The figure shows three views and two pictorial views of one solid part (mm, origin at its lowest corner). Answer the questions. Coordinates: 2 decimals unless noted, no trailing zeros. Loops run counter-clockwise (first coordinate to the right, second up) from the corner with the lowest first, then second, coordinate; pieces in that order, holes last. Notation, with made-up numbers: M 11.25,36 L 15.25,36 A7 ccw 15.25,45 Z; hole C 51.5,45.25 d4. An arc over 180 degrees is marked long. One line per item, written item: value. Start each with the question number.
1. The part is cut by section D-D (y = 4). Write down the section's boundary in (x, z) (1 decimal).
2. Consider probe 1 along Z at (x, y) = (36.5, 9.5); probe 2 along Z at (x, y) = (44, 1.5); probe 3 along Y at (x, z) = (46, 16.75). Determine where each line is inside the solid, lowest interval first.
3. The part is cut by section A-A (z = 7.5). Write down the section's boundary in (x, y).
4. Determine the mould class of the marked faces 1, 2, 3 and 4 for opening direction Z: +Z half, -Z half, draft (parallel to the pull), parting line (faces both ways), or undercut.
5. The part is cut by section B-B (x = 21.5). Write down the section's boundary in (y, z).
6. Flat-ended cylindrical pins translate along their axes: pin 1 (4 mm diameter, centred on x = 43.97, z = 7.5, fed in from +Y); pin 2 (5 mm diameter, centred on y = 8, z = 21, fed in from -X); pin 3 (2 mm diameter, centred on y = 3, z = 25.5, fed in from -X) (1 decimal); pin 4 (2.5 mm diameter, centred on x = 37.67, z = 7.5, fed in from -Y). Find the tip coordinate at first contact, or state that the pin passes through.
7. The part is cut by section C-C (z = 12.5). Write down the section's boundary in (x, y).
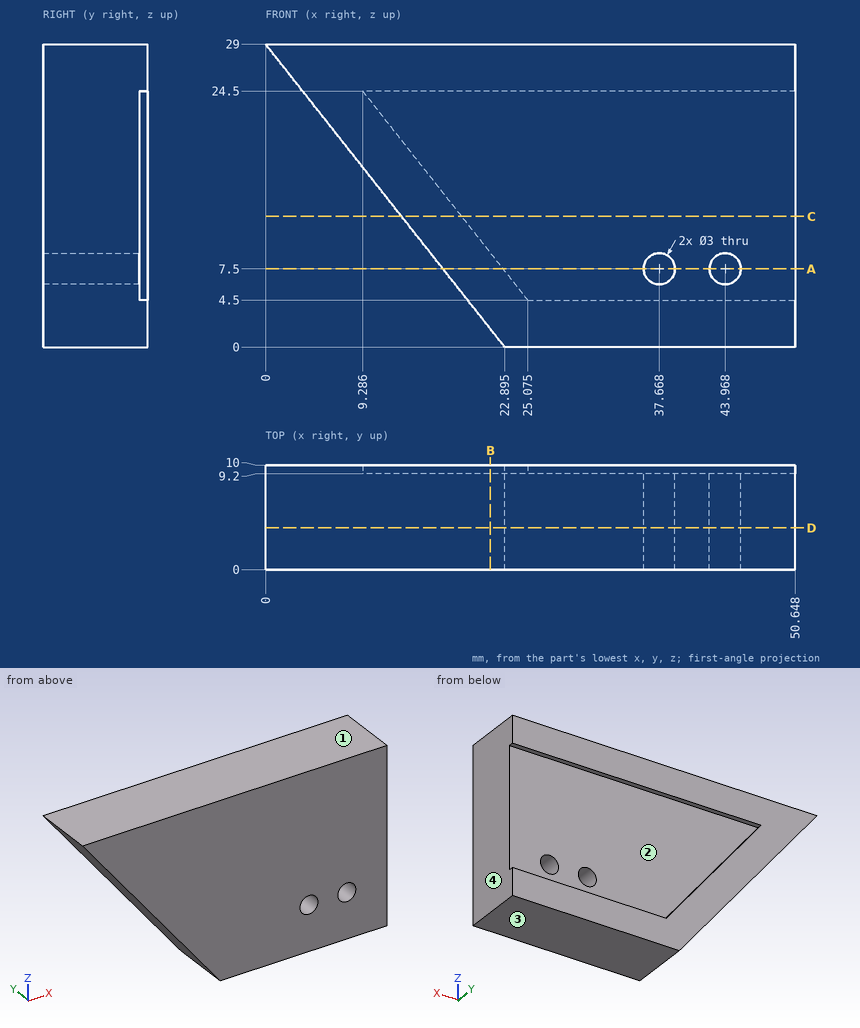
Answer block:
1. outline: M 0,29 L 22.9,0 L 50.6,0 L 50.6,29 Z; hole C 37.7,7.5 d3; hole C 44,7.5 d3
2. probe 1: z = 0 to 4.5, 24.5 to 29
2. probe 2: z = 0 to 6, 9 to 29
2. probe 3: y = 0 to 9.2
3. outline: M 16.97,0 L 36.17,0 L 36.17,9.2 L 22.71,9.2 L 22.71,10 L 16.97,10 Z; M 39.17,0 L 42.47,0 L 42.47,9.2 L 39.17,9.2 Z; M 45.47,0 L 50.65,0 L 50.65,9.2 L 45.47,9.2 Z
4. face 1: +Z half
4. face 2: undercut
4. face 3: -Z half
4. face 4: draft
5. outline: M 0,1.77 L 10,1.77 L 10,9.03 L 9.2,9.03 L 9.2,24.5 L 10,24.5 L 10,29 L 0,29 Z
6. pin 1: stops at y = 9.2
6. pin 2: stops at x = 4.34
6. pin 3: stops at x = 2
6. pin 4: passes through
7. outline: M 13.03,0 L 50.65,0 L 50.65,9.2 L 18.76,9.2 L 18.76,10 L 13.03,10 Z
